Print and shaded views of the part. All mm, measured from the part's lowest x, y and z. A direction names the side the tool comes from. Coordinates: 2 decimals unless noted, no trailing zeros. Order: outer loops, then holes, each group sorted by start corner. A loop starts at its lowest first (then second) coordinate and runs counter-clockwise, first axis right, second up. Notation, with made-up numbers: (23.25, 59) -> (48.25, 59) arc R28 ccw to (48.25, 98) -> close; hole circle Ø5 at (-10, -10). An arc over 180 degrees is marked (long way). Write item = value, one per line. Start each with the question number.
Q1. Cut at C-C, the plane y = 1.25. List the corners of the cut face in (x, z) (1 decimal).
Q2. Mould opens along X. For the marked faces 1, 2, 3 and 4 say: +X half, -X half, draft (parallel to the pull), parting line (faces both ways), or undercut.
Q3. Cut at A-A, the plane x = 4. List the corners of the cut face in (y, z).
Q4. Wall check: line 1 (Z direction, x = 4, y = 10.25); line 2 (X direction, y = 0.5, z = 7.25); line 3 (X direction, y = 9.25, z = 10.25) (1 decimal). Give the ranges that are in metal, low to high. Write a range as from..to.
Q5. 3-axis set-ups, long thin cutter, end or side, ignore diameter. For the marked faces 5, 6, 7 and 8: which of +Z, -Z, +X, -X, +Y, -Y reach the whole face in a straight line?
Q6. Cut at D-D, the plane z = 11. List the corners of the cut face in (x, y) (1 decimal), plus the area to 3 significant figures.
Q7. Flat gauge pins, fed straight in: pin 1 (5 mm diameter, centred on x = 17, y = 5, fed in from -Z) (1 decimal); pin 2 (6 mm diameter, centred on x = 17, z = 10.5, fed in from -Y); pin 3 (4 mm diameter, centred on x = 12.5, y = 7.5, fed in from -Z). Where does each tip first touch, or does it go through?
Q8. Cut at B-B, the plane z = 4. List the corners of the cut face in (x, y) (1 decimal).
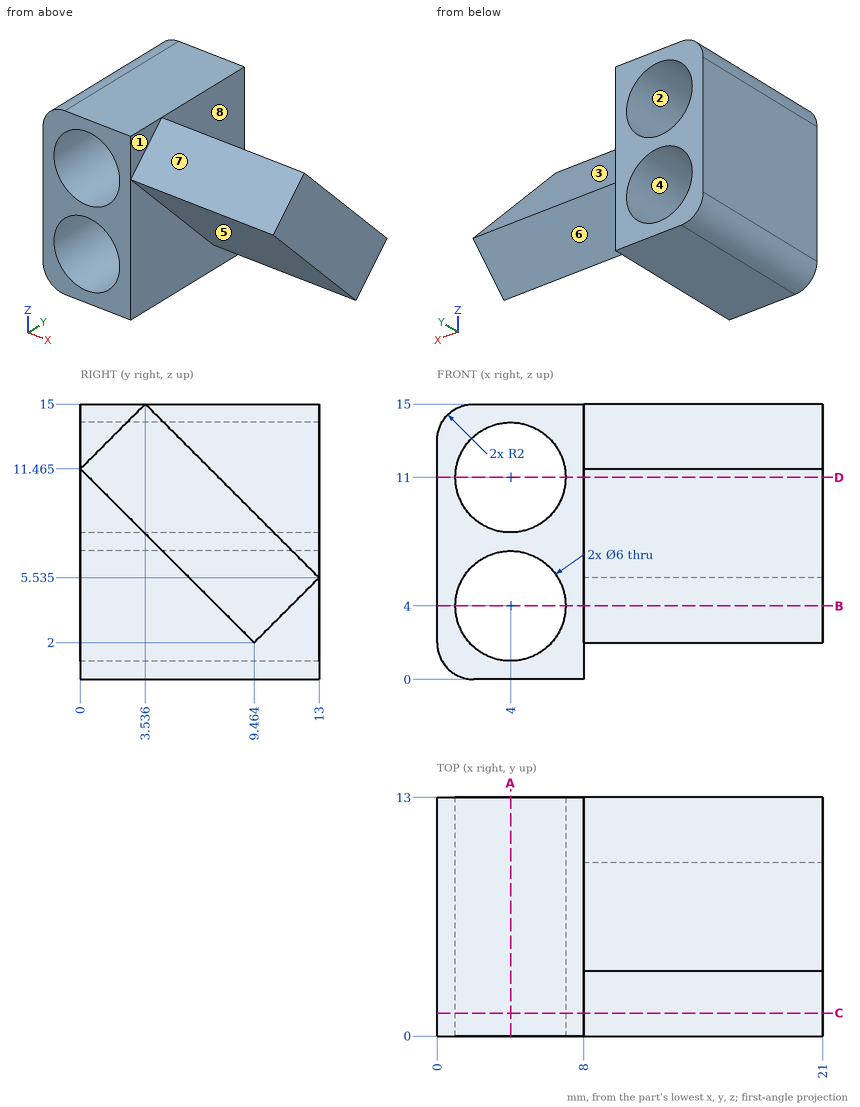
Here are the results:
q1.outline = (0, 2) arc R2 ccw to (2, 0) -> (8, 0) -> (8, 10.2) -> (21, 10.2) -> (21, 12.7) -> (8, 12.7) -> (8, 15) -> (2, 15) arc R2 ccw to (0, 13) -> close; hole circle Ø6 at (4, 4); hole circle Ø6 at (4, 11)
q2.face_1 = +X half
q2.face_2 = undercut
q2.face_3 = draft
q2.face_4 = undercut
q3.outline = (0, 0) -> (13, 0) -> (13, 1) -> (0, 1) -> close; (0, 7) -> (13, 7) -> (13, 8) -> (0, 8) -> close; (0, 14) -> (13, 14) -> (13, 15) -> (0, 15) -> close
q4.line_1 = 0..1, 7..8, 14..15
q4.line_2 = 0..8
q4.line_3 = 0..1.1, 6.9..8
q5.face_5 = -Z, +X, -Y
q5.face_6 = -Z, +X, +Y
q5.face_7 = +Z, +X, -Y
q5.face_8 = +Z, +X, +Y
q6.outline = (0, 0) -> (1, 0) -> (1, 13) -> (0, 13) -> close; (7, 0) -> (8, 0) -> (8, 0.5) -> (21, 0.5) -> (21, 7.5) -> (8, 7.5) -> (8, 13) -> (7, 13) -> close
q6.area = 118 mm²
q7.pin_1 = 4
q7.pin_2 = 0
q7.pin_3 = 2
q8.outline = (0, 0) -> (1, 0) -> (1, 13) -> (0, 13) -> close; (7, 0) -> (8, 0) -> (8, 7.5) -> (21, 7.5) -> (21, 11.5) -> (8, 11.5) -> (8, 13) -> (7, 13) -> close
